Check sheet for the modelled part. Datum: model origin and axes. Units: mm. A direction names the side the tool comes from. Round coordinates to 2 decimals unless told otherwise and drop trailing zeros. Order: outer loops, then holes, each group sorted by start corner. A loop starts at its lowest first (then second) coordinate and runs counter-clockwise, first axis right, second up.
Q1. Depth check by flat-ended pin: P1, Ø1.3, axis at y = 13, z = -26, coming from the -X side; P2, Ø4.5, axis at y = 4.5, z = -27, coming from the +X side; P3, Ø1, axis at y = 4, z = -21, coming from the -X side. Enter the tip coordinate at first touch or a pass-through.
Q2. Cross-section at A-A on z = -5. Record the cut outline in (x, y), then the cut area to 3 significant figures.
Q3. Scan lines: probe 1 along Z at (x, y) = (1.5, 2.5); probe 2 along Z at (x, y) = (-5.5, 20); probe 3 along Z at (x, y) = (-5, 6). Record each from-to range of solid material in increasing order.
Q4. Cross-section at B-B on x = 6. Record the cut outline in (y, z), then the cut area to 3 significant figures.
Q5. Cross-section at C-C on x = -7. Record the cut outline in (y, z).
Q6. Cross-section at D-D on x = 21. Record the cut outline in (y, z), then the cut area to 3 significant figures.
Q7. Set-up check for faces 4 (the flat face through (-10, 17, 35)), 5 (the flat face through (16.5, 17, 16)), 6 (the flat face through (6, 21, -28)), 7 (the flat face through (-23.3, 17, -31)), 8 (the flat face through (-13, 17, 32)): record each of +Z, -Z, +X, -X, +Y, -Y from which the full face is reachable in a straight line by a thin tool's end or side.
Q8. Mould release check, pull along Y, two halves, no side actions. Record for faces 1 (the flat face through (-8, 34, 21)), 2 (the flat face through (6, 13, -28)), 3 (the flat face through (1, 17, -27)): +Y half, -Y half, draft (parallel to the pull), parting line (faces both ways), or undercut.
from build123d import *

# Parameters (mm, degrees)
BOSS_EXTRUDE1_DEPTH = 34
BOSS_EXTRUDE3_DEPTH = 12
CUT_EXTRUDE1_DEPTH  = 14.407172


with BuildPart() as part:
    # Sketch1 → Boss-Extrude1 (new body)
    with BuildSketch(Plane(origin=(0, 0, 0), x_dir=(1, 0, 0), z_dir=(0, 1, 0))):
        with BuildLine():
            Line((14.551632211, 16.5), (16.5, 16.5))
            Line((16.5, 16.5), (16.5, 14.551632211))
            ThreePointArc((16.5, 14.551632211), (22, 0), (16.5, -14.551632211))
            Line((16.5, -14.551632211), (16.5, -16.5))
            Line((16.5, -16.5), (14.551632211, -16.5))
            ThreePointArc((14.551632211, -16.5), (0, -22), (-14.551632211, -16.5))
            Line((-14.551632211, -16.5), (-16.5, -16.5))
            Line((-16.5, -16.5), (-16.5, -14.551632211))
            ThreePointArc((-16.5, -14.551632211), (-22, 0), (-16.5, 14.551632211))
            Line((-16.5, 14.551632211), (-16.5, 16.5))
            Line((-16.5, 16.5), (-14.551632211, 16.5))
            ThreePointArc((-14.551632211, 16.5), (-8.243992543, 20.396974946), (-1, 21.977260976))
            Line((-1, 21.977260976), (-1, 32))
            Line((-1, 32), (-23.299524673, 32))
            Line((-23.299524673, 32), (-23.299524673, 29))
            Line((-23.299524673, 29), (-4, 29))
            Line((-4, 29), (-4, 24.677925359))
            ThreePointArc((-4, 24.677925359), (-10.225195, 22.813272172), (-15.759494281, 19.407172386))
            ThreePointArc((-15.759494281, 19.407172386), (-18.621320344, 18.621320344), (-19.407172386, 15.759494281))
            ThreePointArc((-19.407172386, 15.759494281), (-25, 0), (-19.407172386, -15.759494281))
            ThreePointArc((-19.407172386, -15.759494281), (-18.621320344, -18.621320344), (-15.759494281, -19.407172386))
            ThreePointArc((-15.759494281, -19.407172386), (-9.7623033, -23.015156621), (-3, -24.819347292))
            Line((-3, -24.819347292), (-3, -32))
            Line((-3, -32), (-23.299524673, -32))
            Line((-23.299524673, -32), (-23.299524673, -35))
            Line((-23.299524673, -35), (4, -35))
            Line((4, -35), (15.759494281, -19.407172386))
            ThreePointArc((15.759494281, -19.407172386), (18.621320344, -18.621320344), (19.407172386, -15.759494281))
            ThreePointArc((19.407172386, -15.759494281), (25, 0), (19.407172386, 15.759494281))
            ThreePointArc((19.407172386, 15.759494281), (18.621320344, 18.621320344), (15.759494281, 19.407172386))
            Line((15.759494281, 19.407172386), (5, 32))
            Line((5, 32), (1, 32))
            Line((1, 32), (1, 21.977260976))
            ThreePointArc((1, 21.977260976), (8.243992543, 20.396974946), (14.551632211, 16.5))
        make_face()
        with BuildLine():
            ThreePointArc((0, -25), (4.613293609, -24.570663851), (9.068134921, -23.297401766))
            Line((9.068134921, -23.297401766), (2.504979303, -32))
            Line((2.504979303, -32), (0, -32))
            Line((0, -32), (0, -25))
        make_face(mode=Mode.SUBTRACT)
        with BuildLine():
            ThreePointArc((8.223751321, 23.608683026), (6.135213434, 24.235493725), (4, 24.677925359))
            Line((4, 24.677925359), (4, 28.552128404))
            Line((4, 28.552128404), (8.223751321, 23.608683026))
        make_face(mode=Mode.SUBTRACT)
    extrude(amount=BOSS_EXTRUDE1_DEPTH)

    # Sketch6 → Boss-Extrude3 (add)
    with BuildSketch(Plane(origin=(0, 23, 0), x_dir=(0, 0, -1), z_dir=(0, -1, 0))):
        Polygon((30.717367885, 3.963704263), (22.785433959, 3.963704263), (22.785433959, 10.604126234), align=None)
    extrude(amount=BOSS_EXTRUDE3_DEPTH)

    # Sketch3 → Cut-Extrude1 (cut)
    with BuildSketch(Plane.ZY.offset(-19.407172386)):
        with BuildLine():
            ThreePointArc((-23, 17), (-24.171572875, 19.828427125), (-27, 21))
            Line((-27, 21), (-27, 13))
            ThreePointArc((-27, 13), (-24.171572875, 14.171572875), (-23, 17))
        make_face()
        with BuildLine():
            Line((-27, 13), (-27, 21))
            ThreePointArc((-27, 21), (-31, 17), (-27, 13))
        make_face()
        with BuildLine():
            Line((-27, 21), (-32, 21))
            Line((-32, 21), (-32, 13))
            Line((-32, 13), (-27, 13))
            ThreePointArc((-27, 13), (-31, 17), (-27, 21))
        make_face()
    extrude(amount=CUT_EXTRUDE1_DEPTH, mode=Mode.SUBTRACT)


solid = part.part
Results found:
1. P1: stops at x = -4
1. P2: stops at x = 11.19
1. P3: stops at x = -14.31
2. outline: (-24.49, 0) - (-21.42, 0) - (-21.42, 34) - (-24.49, 34) - close; (21.42, 0) - (24.49, 0) - (24.49, 34) - (21.42, 34) - close
2. area: 209 mm2
3. probe 1: z = -32 to -21.95, 21.95 to 24.95, 32 to 35
3. probe 2: z = -32 to -29, -24.39 to -21.3, 21.3 to 24.39, 32 to 35
3. probe 3: z = -32 to -29, -24.49 to -21.42, 21.42 to 24.49, 32 to 35
4. outline: (0, -30.83) - (13, -30.83) - (13, -27) arc R4 cw to (21, -27) - (21, -30.83) - (34, -30.83) - (34, -26.21) - (23, -26.21) - (23, -24.27) - (34, -24.27) - (34, -21.17) - (0, -21.17) - (0, -24.27) - (11, -24.27) - (11, -26.21) - (0, -26.21) - close; (0, 21.17) - (34, 21.17) - (34, 24.27) - (0, 24.27) - close; (0, 27.37) - (34, 27.37) - (34, 32.35) - (0, 32.35) - close
4. area: 505 mm2
5. outline: (0, -32) - (34, -32) - (34, -29) - (0, -29) - close; (0, -24) - (34, -24) - (34, -20.86) - (0, -20.86) - close; (0, 20.86) - (34, 20.86) - (34, 24) - (0, 24) - close; (0, 32) - (34, 32) - (34, 35) - (0, 35) - close
6. outline: (0, -13.56) - (34, -13.56) - (34, -6.56) - (0, -6.56) - close; (0, 6.56) - (34, 6.56) - (34, 13.56) - (0, 13.56) - close
6. area: 476 mm2
7. face 4: +Z, +X, -X, +Y, -Y
7. face 5: +Y, -Y
7. face 6: -Z, +X
7. face 7: -Z, -X, +Y, -Y
7. face 8: -X, +Y, -Y
8. face 1: +Y half
8. face 2: undercut
8. face 3: draft
